Source: three-view drawing plus pictorial views. Frame: mm from the lowest corner of the part. A direction names the side the tool comes from. Coordinates: 2 decimals unless noted, no trailing zeros. Write each loop counter-clockwise with the first axis right and the second up, starting at its lowest first coordinate (ties: lowest second). Pieces come first, ordered by that corner, then holes. Notation, with made-up numbers: (32.5, -26) - (59.5, -26) arc R12 ccw to (59.5, -22) - close; hole circle Ø9 at (66, -33). An arc over 180 degrees is marked (long way). Put each result on its own line as item: value. Start each with the question number.
1. Access query for the marked faces 3 and 4. Directions: +Z, -Z, +X, -X, +Y, -Y. A direction counts if a zero-diameter tool reaches every point of the face in a straight line with its end or side. Return the directions, or none.
2. Pull-direction query (X, two-part tool) for the marked faces 1 and 2; classes: released by +X, released by -X, zero draft, split by the parting line, or undercut.
3. Cut plane A-A, the plane x = 96. Return loops of the section in (y, z), and give its area (3 significant figures).
4. Cut plane C-C, the plane y = 84. Return loops of the section in (x, z) (1 decimal).
5. Line query: line 1 (Y direction, x = 96, z = 0.4); line 2 (Z direction, x = 42.5, y = 71.5). Output: solid intervals per line, ascending.
6. Pin query (flat end, axial travel): pin 1 (8 mm diameter, centred on x = 79, z = 38.5, fed in from +Y) (1 decimal); pin 2 (8 mm diameter, centred on x = 42, z = 26.5, fed in from +Y); pin 3 (1.5 mm diameter, centred on x = 67, z = 19, fed in from -Y). Return the tip coordinate at first contact, or that it passes through.
7. Cut plane D-D, the plane z = 29. Return loops of the section in (x, y) (1 decimal).
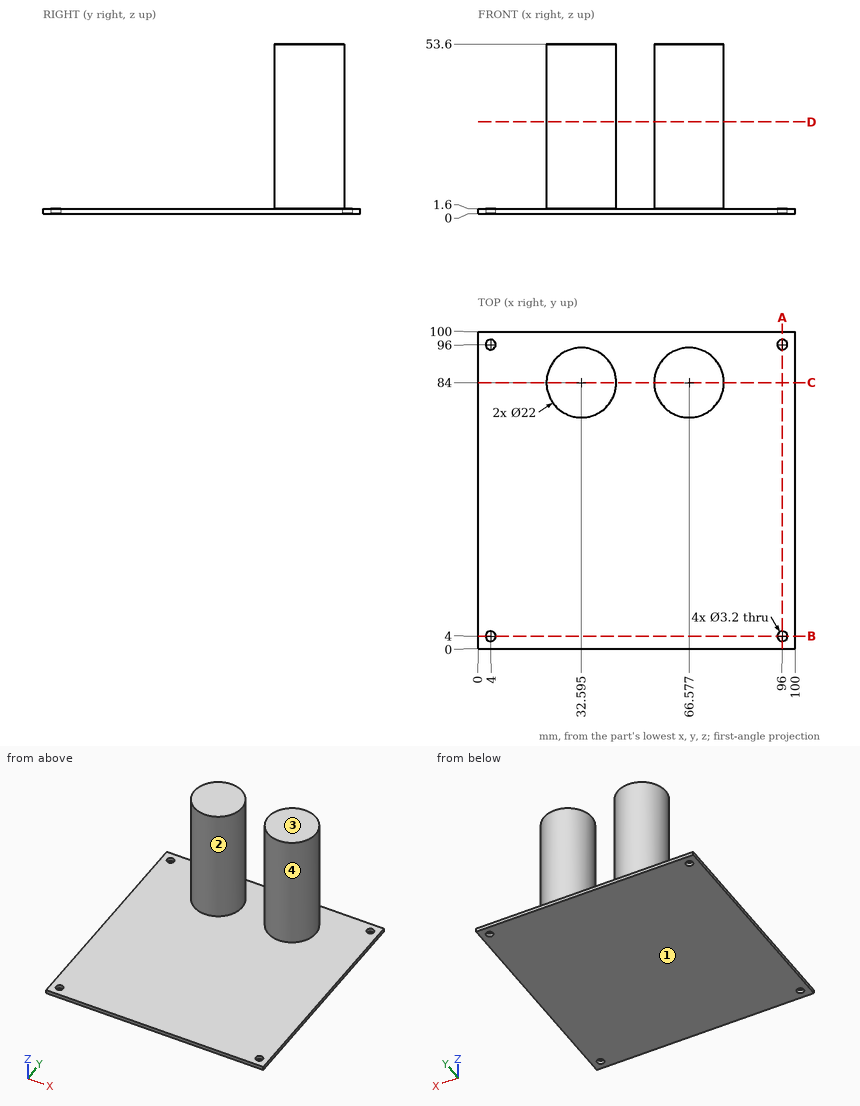
Report:
1. face 3: +Z, +X, -X, +Y, -Y
1. face 4: +Z
2. face 1: zero draft
2. face 2: undercut
3. outline: (0, 0) - (2.4, 0) - (2.4, 1.6) - (0, 1.6) - close; (5.6, 0) - (94.4, 0) - (94.4, 1.6) - (5.6, 1.6) - close; (97.6, 0) - (100, 0) - (100, 1.6) - (97.6, 1.6) - close
3. area: 150 mm^2
4. outline: (0, 0) - (100, 0) - (100, 1.6) - (77.6, 1.6) - (77.6, 53.6) - (55.6, 53.6) - (55.6, 1.6) - (43.6, 1.6) - (43.6, 53.6) - (21.6, 53.6) - (21.6, 1.6) - (0, 1.6) - close
5. line 1: y = 0 to 2.4, 5.6 to 94.4, 97.6 to 100
5. line 2: z = 0 to 1.6
6. pin 1: stops at y = 91.1
6. pin 2: stops at y = 93.58
6. pin 3: stops at y = 73
7. outline: circle Ø22 at (32.6, 84); circle Ø22 at (66.6, 84)
